For this review, take the finished solid that the model builds, in its own axes (mm). Face numbers are marked on the shaded views. A direction names the side the tool comes from. Coordinates: 2 decimals unless noted, no trailing zeros. Loops run counter-clockwise (first coordinate to the right, second up) from the corner with the lowest first, then second, coordinate; pieces in that order, holes last. Notation, with made-up numbers: (35.5, -32.5) -> (67.5, -32.5) arc R27 ccw to (67.5, -1.5) -> close; hole circle Ø7 at (-40, 36). An arc over 180 degrees is marked (long way). Answer in a Markdown table with one row per item.
from build123d import *

# Parameters (mm, degrees)
F0_W     = 203.2
F0_H     = 127
F1_DEPTH = 127
F3_DEPTH = 101.6
F4_SIZE2 = 101.6
F4_SIZE  = 76.2
F5_R     = 5.08
F6_R     = 15.24
F7_DEPTH = 25.4
F8_R     = 15.24
F9_DEPTH = 127


with BuildPart() as f1:
    # F0 (on Front) → F1 (new body)
    with BuildSketch(Plane.XZ):
        with Locations((-4.1312798858, 3.5229725738)):
            Rectangle(F0_W, F0_H)
    extrude(amount=F1_DEPTH)

    # F2 (on face) → F3 (cut)
    with BuildSketch(Plane.XZ.offset(127)):
        Polygon((97.4687201142, 67.0229725738), (-4.1312798858, 67.0229725738), (-4.1312798858, 3.5229718778), (-42.2312798858, 3.5229718778), (-42.2312798858, -59.9770274262), (97.4687201142, -59.9770274262), align=None)
    extrude(amount=-F3_DEPTH, mode=Mode.SUBTRACT)

    # F4
    f4_edges = [f1.edges().sort_by_distance(p)[0] for p in [
        (97.46872, -12.7, 67.022973),
    ]]
    f4_side = f1.faces().sort_by_distance((-37.997947, -55.033333, 67.022973))[0]
    chamfer(f4_edges, length=F4_SIZE, length2=F4_SIZE2, reference=f4_side)

    # F5
    f5_edges = [f1.edges().sort_by_distance(p)[0] for p in [
        (-42.23128, 0, 67.022973),
        (21.26872, -12.7, 67.022973),
        (-105.73128, -63.5, 67.022973),
        (8.56872, -25.4, 67.022973),
        (-54.93128, -127, 67.022973),
        (-4.13128, -76.2, 67.022973),
        (-73.98128, -127, -59.977027),
        (-105.73128, -127, 3.522973),
        (-4.13128, -127, 35.272972),
        (-23.18128, -127, 3.522972),
        (-42.23128, -127, -28.227028),
        (-4.13128, -76.2, 3.522972),
        (-4.13128, -25.4, 35.272972),
        (-42.23128, -76.2, 3.522972),
        (-42.23128, -76.2, -59.977027),
        (-42.23128, -25.4, -28.227028),
        (97.46872, -25.4, -47.277027),
        (59.36872, -25.4, 16.222973),
        (27.61872, -25.4, -59.977027),
        (-23.18128, -25.4, 3.522972),
        (59.36872, 0, 16.222973),
        (97.46872, -12.7, -34.577027),
        (97.46872, 0, -47.277027),
        (97.46872, -12.7, -59.977027),
        (-105.73128, -63.5, -59.977027),
        (-105.73128, 0, 3.522973),
        (-4.13128, 0, -59.977027),
    ]]
    fillet(f5_edges, radius=F5_R)

    # F6 (on face) → F7 (cut)
    with BuildSketch(Plane.XZ.offset(25.4)):
        with Locations((13.6487201142, -14.2570274262)):
            Circle(F6_R)
    extrude(amount=-F7_DEPTH, mode=Mode.SUBTRACT)

    # F8 (on face) → F9 (cut)
    with BuildSketch(Plane.XY.offset(67.0229725738)):
        with Locations((-73.9812798858, -80.01)):
            Circle(F8_R)
    extrude(amount=-F9_DEPTH, mode=Mode.SUBTRACT)


solid = f1.part
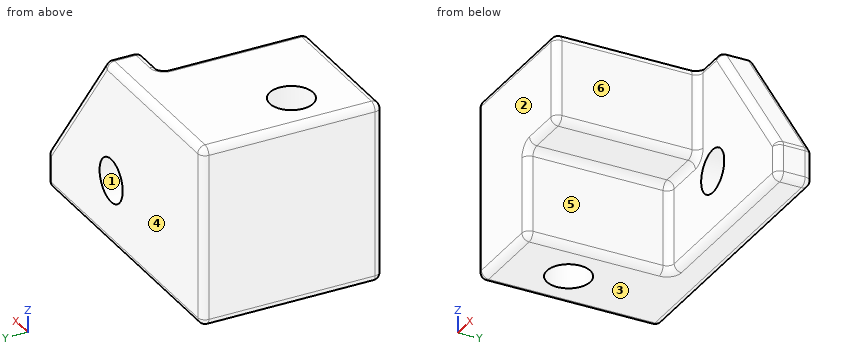
Item 1: For the marked faces 4, 5 and 6, list the 3-axis set-ups (+Z, -Z, +X, -X, +Y, -Y) from which the entire face can be reached by the end or side of a thin tool; tool diameter is ignored.
Worked answers:
| item | result |
|---|---|
| face 4 | +Z, -Z, +X, -X, +Y |
| face 5 | -Z, +X, -Y |
| face 6 | +Z, -Z, +X, -Y |
Item 2: Take a section at D-D, the plane x = 11. State the section outline as (y, z) points.
Worked answers:
| item | result |
|---|---|
| outline | (-25.4, -54.9) arc R5.08 ccw to (-20.32, -59.98) -> (-5.08, -59.98) arc R5.08 ccw to (0, -54.9) -> (0, -29.27) -> (-25.4, -29.27) -> close; (-25.4, 0.75) -> (0, 0.75) -> (0, 61.94) arc R5.08 ccw to (-5.08, 67.02) -> (-20.32, 67.02) arc R5.08 ccw to (-25.4, 61.94) -> close |
Item 3: Take a section at C-C, the plane x = -22. State the section outline as (y, z) points, and give its area (3 significant figures).
Worked answers:
| item | result |
|---|---|
| outline | (-127, 8.6) arc R5.08 ccw to (-121.92, 3.52) -> (-30.48, 3.52) arc R5.08 cw to (-25.4, -1.56) -> (-25.4, -54.9) arc R5.08 ccw to (-20.32, -59.98) -> (-5.08, -59.98) arc R5.08 ccw to (0, -54.9) -> (0, 61.94) arc R5.08 ccw to (-5.08, 67.02) -> (-121.92, 67.02) arc R5.08 ccw to (-127, 61.94) -> close |
| area | 9,660 mm² |
Item 4: For L1, parallel to Y at x = 78.5, z = -48; L2, parallel to X at y = -114, z = -25; L3, parallel to Y at x = -13.5, z = 8.5, list the stretches that pass through material, from the lowest coordinate up.
Worked answers:
| item | result |
|---|---|
| L1 | -25.4 to 0 |
| L2 | -105.73 to -42.23 |
| L3 | -127 to 0 |
Item 5: Take a section at B-B, the plane z = -49. State the section outline as (x, y) points, and give its area (3 significant figures).
Worked answers:
| item | result |
|---|---|
| outline | (-105.73, -121.92) arc R5.08 ccw to (-100.65, -127) -> (-47.31, -127) arc R5.08 ccw to (-42.23, -121.92) -> (-42.23, -30.48) arc R5.08 cw to (-37.15, -25.4) -> (92.39, -25.4) arc R5.08 ccw to (97.47, -20.32) -> (97.47, -5.08) arc R5.08 ccw to (92.39, 0) -> (-100.65, 0) arc R5.08 ccw to (-105.73, -5.08) -> close; hole circle Ø30.48 at (-73.98, -80.01) |
| area | 10,900 mm² |
Item 6: Take a section at A-A, the plane y = -80.01. State the section outline as (x, z) points, and give its area (3 significant figures).
Worked answers:
| item | result |
|---|---|
| outline | (-105.73, -54.9) arc R5.08 ccw to (-100.65, -59.98) -> (-89.22, -59.98) -> (-89.22, 67.02) -> (-100.65, 67.02) arc R5.08 ccw to (-105.73, 61.94) -> close; (-58.74, -59.98) -> (-47.31, -59.98) arc R5.08 ccw to (-42.23, -54.9) -> (-42.23, -1.56) arc R5.08 cw to (-37.15, 3.52) -> (-9.21, 3.52) arc R5.08 ccw to (-4.13, 8.6) -> (-4.13, 61.94) arc R5.08 ccw to (-9.21, 67.02) -> (-58.74, 67.02) -> close |
| area | 6,590 mm² |
Item 7: The part is to be moulded in two halves that separate along Z. For the marked faces 1, 2 and 3, say which applies: +Z half, -Z half, draft (parallel to the pull), parting line (faces both ways), or undercut.
Worked answers:
| item | result |
|---|---|
| face 1 | undercut |
| face 2 | draft |
| face 3 | -Z half |
Item 8: Insertion check: pin 1 (10 mm diameter, centred on x = 6.5, z = -29, fed in from +Y); pin 2 (8 mm diameter, centred on x = -35, y = -77, fed in from -Z); pin 3 (8 mm diameter, centred on x = -29.5, z = -33, fed in from -Y). Each pin has a flat end and moves straight along its axis. Give the tip position at first contact, or say it passes through.
Worked answers:
| item | result |
|---|---|
| pin 1 | y = 0 |
| pin 2 | z = 3.17 |
| pin 3 | y = -25.4 |
